Job drawing, mm, ordinate dimensions from the low corner. One solid piece. A direction names the side the tool comes from. Give positions to 0.01 mm unless a question says otherwise; leave off trailing zeros. Order: outer loops, then holes, each group sorted by start corner. A loop starts at its lowest first (then second) coordinate and runs counter-clockwise, first axis right, second up. Notation, with made-up numbers: (3, -5) -> (8, -5) arc R21 cw to (8, 2) -> close; hole circle Ø2 at (48.25, 27). An arc over 180 degrees is marked (long way). Write item = value, one per line. Start each with the question number.
(1) Probe line 1 along Y through (x, z) = (5, 40.6) (1 decimal); line 2 along Y through (x, z) = (25, 19); line 3 along Z through (x, y) = (35.5, 21). List the from-to ranges inside material, lowest first. Write a range as from..to.
(2) Flat gauge pins, fed straight in: pin 1 (4.5 mm diameter, centred on x = 35.005, y = 8.195, fed in from -Z); pin 2 (11 mm diameter, centred on x = 28, z = 10.5, fed in from +Y); pin 3 (4.5 mm diameter, centred on x = 35.005, y = 32.195, fed in from +Z). Where does each tip first touch, or does it go through?
(3) Saw through at C-C, the plane x = 5. List the corners of the cut face in (y, z) (1 decimal), then the cut area to 3 significant figures.
(4) Which spindle directions (+Z, -Z, +X, -X, +Y, -Y) get a long thin tool onto all of the face, cutting with end or side? Do the marked faces 1 and 2. Say none if no direction does.
(5) Saw through at B-B, the plane x = 15. List the corners of the cut face in (y, z) (1 decimal).
(6) Saw through at D-D, the plane y = 24. List the corners of the cut face in (x, z) (1 decimal).
(7) Saw through at A-A, the plane z = 27. List the corners of the cut face in (x, y) (1 decimal).
(8) Two-plate mould, pull along Y, no slides. Class the marked faces 3, 4 and 5: pulls with the +Y half, pulls with the -Y half, needs draft (parallel to the pull), parting line crosses it, or undercut.
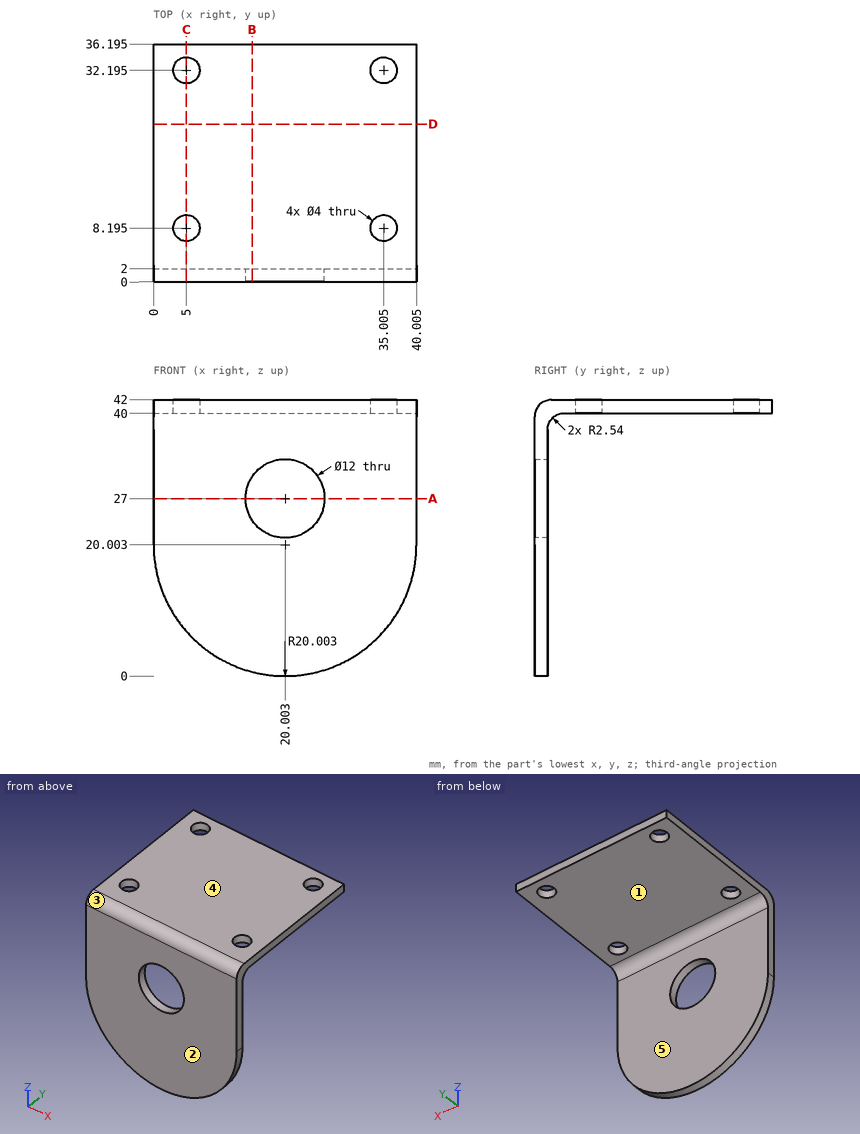
Results list:
q1.line_1 = 0.3..6.2, 10.2..30.2, 34.2..36.2
q1.line_2 = 0..2
q1.line_3 = 40..42
q2.pin_1 = 40
q2.pin_2 = 2
q2.pin_3 = 42
q3.outline = (0, 6.8) -> (2, 6.8) -> (2, 37.5) arc R2.5 cw to (4.5, 40) -> (6.2, 40) -> (6.2, 42) -> (2.5, 42) arc R2.5 ccw to (0, 39.5) -> close; (10.2, 40) -> (30.2, 40) -> (30.2, 42) -> (10.2, 42) -> close; (34.2, 40) -> (36.2, 40) -> (36.2, 42) -> (34.2, 42) -> close
q3.area = 123 mm^2
q4.face_1 = -Z, +X, -X, +Y
q4.face_2 = +Z, -Z, +X, -X, -Y
q5.outline = (0, 0.6) -> (2, 0.6) -> (2, 23.7) -> (0, 23.7) -> close; (0, 30.3) -> (2, 30.3) -> (2, 37.5) arc R2.5 cw to (4.5, 40) -> (36.2, 40) -> (36.2, 42) -> (2.5, 42) arc R2.5 ccw to (0, 39.5) -> close
q6.outline = (0, 40) -> (40, 40) -> (40, 42) -> (0, 42) -> close
q7.outline = (0, 0) -> (14, 0) -> (14, 2) -> (0, 2) -> close; (26, 0) -> (40, 0) -> (40, 2) -> (26, 2) -> close
q8.face_3 = pulls with the -Y half
q8.face_4 = needs draft
q8.face_5 = pulls with the +Y half
